Input: part model. Units: mm. Frame: model coordinates. Give positions to 0.01 mm unless a question says otherwise; leave off trailing zeros. Order: outer loops, then holes, each group sorted by start corner. A loop starts at its lowest first (then second) coordinate and runs counter-clockwise, first axis right, second up. Notation, with made-up numbers: M 72.25,-22.5 L 125.25,-22.5 A10 cw 125.25,-9.5 Z; hole C -7.5,61.25 d11. An arc over 180 degrees is marked long. Use a Markdown table: item, result.
from build123d import *

# Parameters (mm, degrees)
FILLET1_R = 3
FILLET2_R = 1
FILLET3_R = 0.5


with BuildPart() as part:
    # Sketch1 → Revolve1 (revolve)
    with BuildSketch(Plane.XY, mode=Mode.PRIVATE) as revolve1_sk:
        Polygon((0, 0), (3.5, 0), (3.5, 3), (3, 3), (3, 7), (2, 7), (2, 18), (3, 18), (3, 25), (0, 25), align=None)
    revolve(revolve1_sk.sketch.rotate(Axis((0, 25, 0), (0, -1, 0)), 180), axis=Axis((0, 25, 0), (0, -1, 0)))

    # Fillet1
    fillet1_edges = [part.edges().sort_by_distance(p)[0] for p in [
        (3, 25, 0),
    ]]
    fillet(fillet1_edges, radius=FILLET1_R)

    # Fillet2
    fillet2_edges = [part.edges().sort_by_distance(p)[0] for p in [
        (2, 18, 0),
        (2, 7, 0),
    ]]
    fillet(fillet2_edges, radius=FILLET2_R - 0.0001)  # a hair under: the kernel refuses the full size

    # Fillet3
    fillet3_edges = [part.edges().sort_by_distance(p)[0] for p in [
        (3, 3, 0),
    ]]
    fillet(fillet3_edges, radius=FILLET3_R - 0.0001)  # a hair under: the kernel refuses the full size

    # Sketch2 → Cut-Revolve1 (revolve, cut)
    with BuildSketch(Plane.XY, mode=Mode.PRIVATE) as cut_revolve1_sk:
        with BuildLine():
            Line((0, 1.5), (0, 0))
            Line((0, 0), (1.5, 0))
            ThreePointArc((1.5, 0), (1.060660172, 1.060660172), (0, 1.5))
        make_face()
    revolve(cut_revolve1_sk.sketch.rotate(Axis((0, 1.5, 0), (0, -1, 0)), 180), axis=Axis((0, 1.5, 0), (0, -1, 0)), mode=Mode.SUBTRACT)


solid = part.part
1) Material intervals for line 1 (Z direction, x = -2, y = 23); line 2 (X direction, y = 21, z = 1); line 3 (X direction, y = 21.25, z = 1.5), sorted ascending. Write a range as from..to.
Response values:
| item | result |
|---|---|
| line 1 | z = -2..2 |
| line 2 | x = -2.83..2.83 |
| line 3 | x = -2.6..2.6 |
2) First-contact query: pin 1 Ø2 at (x, z) = (-0.5, -1) entering from +Y; pin 2 Ø2 at (y, z) = (19, 2) entering from -X. Flat tips, straight axial feed; report the tip coordinate or a pass-through.
Response values:
| item | result |
|---|---|
| pin 1 | stops at y = 25 |
| pin 2 | stops at x = -2.83 |
3) Mould query, pull axis Y, two halves, no side actions, for faces 1 (the face through (0, 13, 2)), 2 (the face through (0, 0, 2)), 3 (the face through (-3.233, 1.521, 1.341)). Classes: released by +Y, released by -Y, zero draft, split by the parting line, or undercut.
Response values:
| item | result |
|---|---|
| face 1 | undercut |
| face 2 | released by -Y |
| face 3 | zero draft |
4) Cut plane C-C on y = 16.25. Return loops of the section in (x, z), and give its area (3 significant figures).
Response values:
| item | result |
|---|---|
| outline | C 0,0 d4 |
| area | 12.6 mm² |
